Here's how the part is built. I have some questions about the finished solid (model axes, mm). Face numbers are marked on the shaded views. A direction names the side the tool comes from. Coordinates: 2 decimals unless noted, no trailing zeros. Order: outer loops, then holes, each group sorted by start corner. A loop starts at its lowest first (then second) coordinate and runs counter-clockwise, first axis right, second up. Notation, with made-up numbers: (87.5, 37.5) - (106.5, 37.5) arc R18 ccw to (106.5, 48.5) - close; hole circle Ø3 at (-34.5, 53.5). An arc over 180 degrees is marked (long way). Answer as CSV lines item,"result". Start each with the question number.
Q1. Suppose I cut it at A-A (x = 0). Please give me the cut outline in (y, z), then the cut area to 3 significant figures.
Q2. Suppose I cut it at C-C (z = 1). Please give me the cut outline in (x, y), then the cut area to 3 significant figures.
Q3. Suppose I cut it at B-B (y = 0.9). Please give me the cut outline in (x, z).
Q4. Suppose I cut it at D-D (z = -0.5). Please give me the cut outline in (x, y).
Q5. For pin 1 Ø1.6 at (x, y) = (0, -1) entering from -Z; pin 2 Ø1.6 at (x, y) = (1.5, -1) entering from +Z; pin 3 Ø2 at (x, z) = (0, 5) entering from +Y, each with a flat end and sliding along its axis, tell me the tip position at first contact or that it passes through.
Q6. For the marked faces 1 and 2, which set-ups out of +Z, -Z, +X, -X, +Y, -Y let a thin tool reach every point of the face, with its end or its side?
Q7. I need wall thicknesses on line 1 (Y direction, x = -1.35, z = -2) (3 decimals); line 2 (X direction, y = -2.5, z = -0.25); line 3 (Y direction, x = 0, z = 1.5). Which ranges of each line are inside material? Lowest first, please.
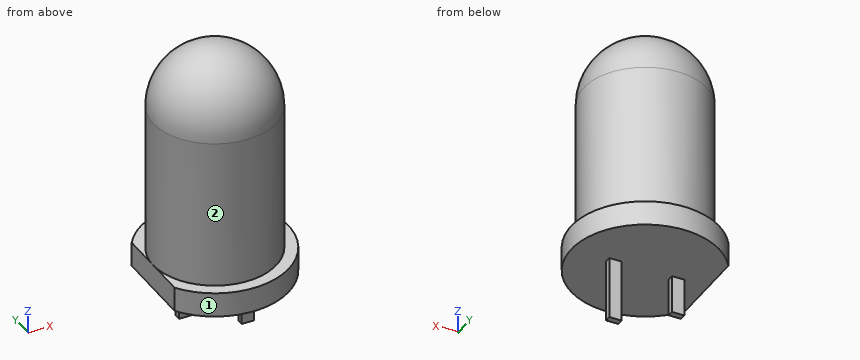
from build123d import *

# Parameters (mm, degrees)
ESBO_O1_R                = 2.5
RESSALTO_EXTRUS_O1_DEPTH = 8.6
RESSALTO_EXTRUS_O2_DEPTH = 1
FILETE1_R                = 2.5
ESBO_O3_W                = 0.5
ESBO_O3_H                = 0.25
RESSALTO_EXTRUS_O3_DEPTH = 2.54
ESBO_O4_W                = 0.935535929
ESBO_O4_H                = 0.753626165
CORTE_EXTRUS_O1_DEPTH    = 1


with BuildPart() as part:
    # Esboço1 → Ressalto-extrusão1 (new body)
    with BuildSketch(Plane.XY):
        with Locations(Location((0, 0, 0), (0, 0, 180))):
            Circle(ESBO_O1_R)
    extrude(amount=RESSALTO_EXTRUS_O1_DEPTH)

    # Esboço2 → Ressalto-extrusão2 (add)
    with BuildSketch(Plane(origin=(0, 0, 0), x_dir=(-1, 0, 0), z_dir=(0, 0, -1))):
        with BuildLine():
            Line((2.5, 0), (2.5, 1.658312395))
            ThreePointArc((2.5, 1.658312395), (-3, 0), (2.5, -1.658312395))
            Line((2.5, -1.658312395), (2.5, 0))
        make_face()
    extrude(amount=RESSALTO_EXTRUS_O2_DEPTH)

    # Filete1
    filete1_edges = [part.edges().sort_by_distance(p)[0] for p in [
        (2.5, 0, 8.6),
    ]]
    fillet(filete1_edges, radius=FILETE1_R)

    # Esboço3 → Ressalto-extrusão3 (add)
    with BuildSketch(Plane(origin=(0, 0, -1), x_dir=(-1, 0, 0), z_dir=(0, 0, -1))):
        with Locations((1.27, 0)):
            Rectangle(ESBO_O3_W, ESBO_O3_H)
        with Locations((-1.27, 0)):
            Rectangle(ESBO_O3_W, ESBO_O3_H)
    extrude(amount=RESSALTO_EXTRUS_O3_DEPTH)

    # Esboço4 → Corte-extrusão1 (cut)
    with BuildSketch(Plane(origin=(0, 0, -3.54), x_dir=(-1, 0, 0), z_dir=(0, 0, -1))):
        with Locations((1.289457258, 0.005956527)):
            Rectangle(ESBO_O4_W, ESBO_O4_H)
    extrude(amount=-CORTE_EXTRUS_O1_DEPTH, mode=Mode.SUBTRACT)


solid = part.part
Here are the results:
1,outline,"(-3, -1) - (3, -1) - (3, 0) - (2.5, 0) - (2.5, 6.1) arc R2.5 ccw to (-2.5, 6.1) - (-2.5, 0) - (-3, 0) - close"
1,area,"46.3 mm²"
2,outline,"circle Ø5 at (0, 0)"
2,area,"19.6 mm²"
3,outline,"(-2.5, -1) - (2.86, -1) - (2.86, 0) - (2.33, 0) - (2.33, 6.1) arc R2.33 ccw to (-2.33, 6.1) - (-2.33, 0) - (-2.5, 0) - close"
4,outline,"(-2.5, -1.66) arc R3 ccw (long way) to (-2.5, 1.66) - close"
5,pin 1,"stops at z = -1"
5,pin 2,"stops at z = 8.39"
5,pin 3,"stops at y = 2.5"
6,face 1,"+Z, -Z"
6,face 2,"+Z"
7,line 1,"y = -0.125 to 0.125"
7,line 2,"x = -1.66 to 1.66"
7,line 3,"y = -2.5 to 2.5"
